Here's how the part is built. I have some questions about the finished solid (model axes, mm). Face numbers are marked on the shaded views. A direction names the side the tool comes from. Coordinates: 2 decimals unless noted, no trailing zeros. Loops run counter-clockwise (first coordinate to the right, second up) from the corner with the lowest first, then second, coordinate; pieces in that order, holes last. Notation, with made-up numbers: (10.25, 42) - (23.25, 42) arc R20 cw to (23.25, 78) - close; hole circle Ø8 at (-17, 49.5). An arc over 180 degrees is marked (long way). Use a Markdown table: item, result.
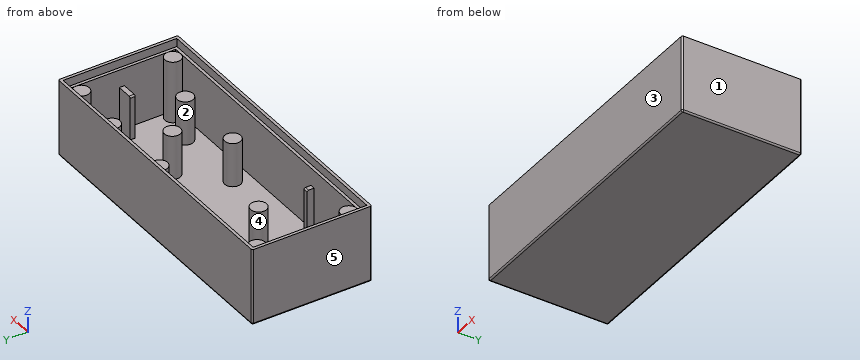
```python
from build123d import *

# Parameters (mm, degrees)
IZIM1_W                     = 100
IZIM1_H                     = 40
Y_KSEKLIK_EKSTR_ZYON1_DEPTH = 25.6
IZIM2_W                     = 96
IZIM2_H                     = 36
KES_EKSTR_ZYON1_DEPTH       = 23.4
IZIM5_R                     = 2.68
Y_KSEKLIK_EKSTR_ZYON6_DEPTH = 22.42
IZIM6_W                     = 98
IZIM6_H                     = 38
KES_EKSTR_ZYON2_DEPTH       = 2.76
IZIM7_W                     = 5.52
IZIM7_H                     = 1.7
Y_KSEKLIK_EKSTR_ZYON7_DEPTH = 14.7
IZIM8_W                     = 1.6
IZIM8_H                     = 2.3
Y_KSEKLIK_EKSTR_ZYON8_DEPTH = 14.7
IZIM9_R                     = 2.68
Y_KSEKLIK_EKSTR_ZYON9_DEPTH = 14.7
RADYUS1_R                   = 0.5


with BuildPart() as part:
    # Çizim1 → Yükseklik-Ekstrüzyon1 (new body)
    with BuildSketch(Plane.XY):
        with Locations((7.815221761, -0.187165775)):
            Rectangle(IZIM1_W, IZIM1_H)
    extrude(amount=Y_KSEKLIK_EKSTR_ZYON1_DEPTH)

    # Çizim2 → Kes-Ekstrüzyon1 (cut)
    with BuildSketch(Plane.XY.offset(25.6)):
        with Locations((7.815221761, -0.187165775)):
            Rectangle(IZIM2_W, IZIM2_H)
    extrude(amount=-KES_EKSTR_ZYON1_DEPTH, mode=Mode.SUBTRACT)

    # Çizim5 → Yükseklik-Ekstrüzyon6 (add)
    with BuildSketch(Plane.XY.offset(2.2)):
        with Locations(Location((-37.494778239, 15.122834225, 0), (0, 0, 180))):
            Circle(IZIM5_R)
        with Locations(Location((-37.494778239, -15.497165775, 0), (0, 0, 180))):
            Circle(IZIM5_R)
        with Locations(Location((53.125221761, -15.497165775, 0), (0, 0, 180))):
            Circle(IZIM5_R)
        with Locations(Location((53.125221761, 15.122834225, 0), (0, 0, 180))):
            Circle(IZIM5_R)
    extrude(amount=Y_KSEKLIK_EKSTR_ZYON6_DEPTH)

    # Çizim6 → Kes-Ekstrüzyon2 (cut)
    with BuildSketch(Plane.XY.offset(25.6)):
        with Locations((7.815221761, -0.187165775)):
            Rectangle(IZIM6_W, IZIM6_H)
    extrude(amount=-KES_EKSTR_ZYON2_DEPTH, mode=Mode.SUBTRACT)

    # Çizim7 → Yükseklik-Ekstrüzyon7 (add)
    with BuildSketch(Plane.XY.offset(2.2)):
        with Locations((53.055221761, -0.187165775)):
            Rectangle(IZIM7_W, IZIM7_H)
        with Locations((-37.424778239, -0.187165775)):
            Rectangle(IZIM7_W, IZIM7_H)
    extrude(amount=Y_KSEKLIK_EKSTR_ZYON7_DEPTH)

    # Çizim8 → Yükseklik-Ekstrüzyon8 (add)
    with BuildSketch(Plane.XY.offset(2.2)):
        with Locations((-14.684778239, 16.662834225)):
            Rectangle(IZIM8_W, IZIM8_H)
        with Locations((-14.684778239, -17.037165775)):
            Rectangle(IZIM8_W, IZIM8_H)
    extrude(amount=Y_KSEKLIK_EKSTR_ZYON8_DEPTH)

    # Çizim9 → Yükseklik-Ekstrüzyon9 (add)
    with BuildSketch(Plane.XY.offset(2.2)):
        with Locations((42.035221761, 12.052834225)):
            Circle(IZIM9_R)
        with Locations(Location((42.035221761, -12.427165775, 0), (0, 0, 180))):
            Circle(IZIM9_R)
        with Locations((17.555221761, 12.052834225)):
            Circle(IZIM9_R)
        with Locations(Location((17.555221761, -12.427165775, 0), (0, 0, 180))):
            Circle(IZIM9_R)
        with Locations((29.795221761, -0.187165775)):
            Circle(IZIM9_R)
        with Locations((-14.684778239, -0.187165775)):
            Circle(IZIM9_R)
    extrude(amount=Y_KSEKLIK_EKSTR_ZYON9_DEPTH)

    # Radyus1
    radyus1_edges = [part.edges().sort_by_distance(p)[0] for p in [
        (-34.664778239, -0.187165775, 16.9),
        (-14.684778239, 15.512834225, 16.9),
        (-14.684778239, -15.887165775, 16.9),
        (7.815221761, 19.812834225, 0),
        (57.815221761, -0.187165775, 0),
        (7.815221761, -20.187165775, 0),
        (-42.184778239, -0.187165775, 0),
        (-42.184778239, 19.812834225, 12.8),
        (57.815221761, 19.812834225, 12.8),
        (57.815221761, -20.187165775, 12.8),
        (-42.184778239, -20.187165775, 12.8),
        (50.295221761, -0.187165775, 16.9),
    ]]
    fillet(radyus1_edges, radius=RADYUS1_R)


solid = part.part
```
Q1. Which directions (+Z, -Z, +X, -X, +Y, -Y) give clear straight access to the entire face, cutting with the end or side of a thin tool? Please do the marked faces 4 and 5.
Check values:
| item | result |
|---|---|
| face 4 | +Z |
| face 5 | +Z, -Z, -X, +Y, -Y |
Q2. I want a section at B-B, the plane x = -4.5. Write out the boundary of the cut face in (y, z), then the cut area to 3 significant figures.
Check values:
| item | result |
|---|---|
| outline | (-20.19, 0.5) arc R0.5 ccw to (-19.69, 0) - (19.31, 0) arc R0.5 ccw to (19.81, 0.5) - (19.81, 25.6) - (18.81, 25.6) - (18.81, 22.84) - (17.81, 22.84) - (17.81, 2.2) - (-18.19, 2.2) - (-18.19, 22.84) - (-19.19, 22.84) - (-19.19, 25.6) - (-20.19, 25.6) - close |
| area | 176 mm^2 |
Q3. Will these pins go through, and if not, where does the flat tip stop? P1, Ø0.8, axis at x = -14.5, y = 17, coming from the +Z side; P2, Ø11.5, axis at x = -5.5, y = -4, coming from the +Z side.
Check values:
| item | result |
|---|---|
| P1 | z = 16.9 |
| P2 | z = 2.2 |
Q4. I want a section at D-D, the plane z = 14. Give the number of separate pieces and of enclosed holes in the cut face, then the cut area to 3 significant figures.
Check values:
| item | result |
|---|---|
| separate pieces | 11 |
| enclosed holes | 1 |
| area | 796 mm^2 |
Q5. I want a section at C-C, the plane y = -8.5. Write out the boundary of the cut face in (x, z), then the cut area to 3 significant figures.
Check values:
| item | result |
|---|---|
| outline | (-42.18, 0.5) arc R0.5 ccw to (-41.68, 0) - (57.32, 0) arc R0.5 ccw to (57.82, 0.5) - (57.82, 25.6) - (56.82, 25.6) - (56.82, 22.84) - (55.82, 22.84) - (55.82, 2.2) - (-40.18, 2.2) - (-40.18, 22.84) - (-41.18, 22.84) - (-41.18, 25.6) - (-42.18, 25.6) - close |
| area | 308 mm^2 |
Q6. If we mould it in two halves opening along X, with no side actions, what happens to the marked faces 1, 2 and 3? For each: pulls with the +X half, pulls with the -X half, needs draft (parallel to the pull), parting line crosses it, or undercut.
Check values:
| item | result |
|---|---|
| face 1 | pulls with the +X half |
| face 2 | undercut |
| face 3 | needs draft |
Q7. Please list where these lines run through material, in increasing order: L1, parallel to Y at x = 29.5, z = 8.25; L2, parallel to Y at x = 46.5, z = 10.5; L3, parallel to X at y = 8.5, z = 10.5. Write a range as from..to.
Check values:
| item | result |
|---|---|
| L1 | -20.19..-18.19, -2.85..2.48, 17.81..19.81 |
| L2 | -20.19..-18.19, 17.81..19.81 |
| L3 | -42.18..-40.18, 55.82..57.82 |
Q8. I want a section at A-A, the plane z = 18.25. Write out the boundary of the cut face in (x, y).
Check values:
| item | result |
|---|---|
| outline | (-42.18, -19.69) arc R0.5 ccw to (-41.68, -20.19) - (57.32, -20.19) arc R0.5 ccw to (57.82, -19.69) - (57.82, 19.31) arc R0.5 ccw to (57.32, 19.81) - (-41.68, 19.81) arc R0.5 ccw to (-42.18, 19.31) - close; circle Ø5.36 at (-37.49, -15.5); circle Ø5.36 at (-37.49, 15.12); circle Ø5.36 at (53.13, -15.5); circle Ø5.36 at (53.13, 15.12); hole (-40.18, -18.19) - (55.82, -18.19) - (55.82, 17.81) - (-40.18, 17.81) - close |
